For this review, take the finished solid that the model builds, in its own axes (mm). Face numbers are marked on the shaded views. A direction names the side the tool comes from. Round coordinates to 2 decimals unless told otherwise and drop trailing zeros. Write each loop counter-clockwise with the first axis right and the second up, starting at its lowest first coordinate (ties: lowest second). Pieces come first, ordered by that corner, then holes. Notation, with made-up numbers: (40, 81.25) -> (86, 81.25) arc R11 cw to (86, 97.25) -> close; hole circle Ø2 at (30, 9.5). An arc over 180 degrees is marked (long way). Answer in a Markdown table with one row per item. Add a question column.
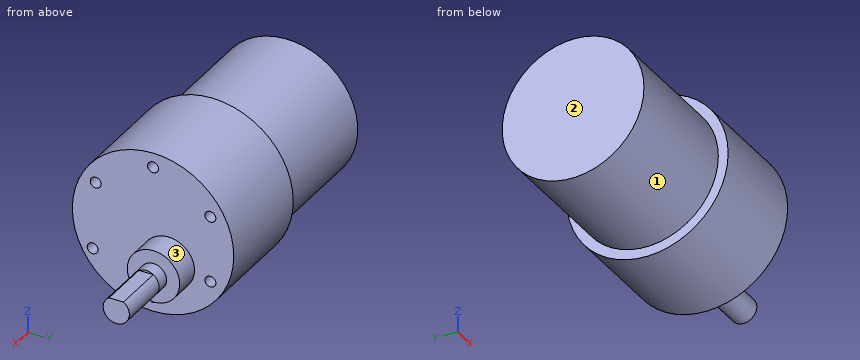
```python
from build123d import *

# Parameters (mm, degrees)
SKETCH061_R             = 16.25
PAD047_DEPTH            = 30
SKETCH062_R             = 18.5
PAD048_DEPTH            = 24
SKETCH063_R             = 1.25
POCKET012_DEPTH         = 4
SKETCH064_R             = 6
PAD049_DEPTH            = 6
SKETCH065_R             = 3
PAD050_DEPTH            = 3
PAD051_DEPTH            = 12
BODY015_ROLL_ANGLE      = -90
BODY015_PLACEMENT_ANGLE = -90


with BuildPart() as part:
    # Sketch061 → Pad047 (new body)
    with BuildSketch(Plane.XY):
        Circle(SKETCH061_R)
    extrude(amount=PAD047_DEPTH)

    # Sketch062 (on Face3 of Pad047) → Pad048 (join)
    with BuildSketch(Plane.XY.offset(30)):
        Circle(SKETCH062_R)
    extrude(amount=PAD048_DEPTH)

    # Sketch063 (on Face5 of Pad048) → Pocket012 (cut)
    with BuildSketch(Plane.XY.offset(54)):
        with Locations((-13.14747, 7.590696)):
            Circle(SKETCH063_R)
        with Locations((-13.14747, -7.590696)):
            Circle(SKETCH063_R)
        with Locations((13.14747, -7.590696)):
            Circle(SKETCH063_R)
        with Locations((0, 15.181391)):
            Circle(SKETCH063_R)
        with Locations((13.853779, 7.998483)):
            Circle(SKETCH063_R)
        with Locations((0, -15.181391)):
            Circle(SKETCH063_R)
    extrude(amount=-POCKET012_DEPTH, mode=Mode.SUBTRACT)

    # Sketch064 (on Face5 of Pocket012) → Pad049 (join)
    with BuildSketch(Plane(origin=(0, 0, 54), x_dir=(0.866025, 0.5, 0), z_dir=(0, 0, 1))):
        with Locations((0, 7)):
            Circle(SKETCH064_R)
    extrude(amount=PAD049_DEPTH)

    # Sketch065 (on Face17 of Pad049) → Pad050 (join)
    with BuildSketch(Plane.XY.offset(60)):
        with Locations((-3.5, 6.062178)):
            Circle(SKETCH065_R)
    extrude(amount=PAD050_DEPTH)

    # Sketch066 (on Face21 of Pad050) → Pad051 (join)
    with BuildSketch(Plane.XY.offset(63)):
        with BuildLine():
            Line((-5.158312, 3.562178), (-1.841688, 3.562178))
            ThreePointArc((-1.841688, 3.562178), (-3.5, 9.062178), (-5.158312, 3.562178))
        make_face()
    extrude(amount=PAD051_DEPTH)


with BuildPart() as part_1:
    # Body015 roll: moved
    add(part.part.rotate(Axis((0, 0, 0), (1, 0, 0)), BODY015_ROLL_ANGLE))


with BuildPart() as part_2:
    # Body015 placement: moved
    add(part_1.part.moved(Location((-199, 213.5, 112))).rotate(Axis((-199, 213.5, 112), (0, 0, 1)), BODY015_PLACEMENT_ANGLE))


solid = part_2.part
```
1. Clearance check with flat-ended pins moving along their axes: pin 1 Ø2 at (y, z) = (201, 119.5) entering from +X; pin 2 Ø2 at (x, z) = (-164, 100.5) entering from -Y; pin 3 Ø1 at (x, y) = (-182.5, 218.5) entering from +Z. State where each tip first meets the part, or that it passes through.
2. For L1, parallel to Z at x = -146.1, y = 213.5; L2, parallel to Z at x = -147, y = 213; L3, parallel to X at y = 201, z = 109.5, list the stretches that pass through material, from the lowest coordinate up. Write a range as [from, to].
3. We need section A-A (z = 101.5). Write out the cut boundary in (x, y).
4. We need section D-D (z = 116). Write out the cut boundary in (x, y).
5. Tool access review of the marked faces 1, 2 and 3: name each direction out of +Z, -Z, +X, -X, +Y, -Y from which nothing blocks a thin tool from reaching the whole face with its end or side.
6. We need section B-B (y = 217). Write out the cut boundary in (x, z), plus the area to 3 significant figures.
7. We need section C-C (x = -172.5). Write out the cut boundary in (y, z).
Response:
| question | item | result |
|---|---|---|
| 1 | pin 1 | x = -145 |
| 1 | pin 2 | y = 198.27 |
| 1 | pin 3 | z = 127.61 |
| 2 | L1 | [93.5, 95.57], [98.07, 125.93], [128.43, 130.5] |
| 2 | L2 | [93.51, 95.67], [97.96, 126.04], [128.33, 130.49] |
| 2 | L3 | [-199, -145] |
| 3 | outline | (-199, 201.1) -> (-169, 201.1) -> (-169, 198.27) -> (-145, 198.27) -> (-145, 212.96) -> (-139, 212.96) -> (-139, 221.04) -> (-145, 221.04) -> (-145, 228.73) -> (-169, 228.73) -> (-169, 225.9) -> (-199, 225.9) -> close |
| 4 | outline | (-199, 197.75) -> (-169, 197.75) -> (-169, 195.44) -> (-145, 195.44) -> (-145, 231.56) -> (-169, 231.56) -> (-169, 229.25) -> (-199, 229.25) -> close |
| 5 | face 1 | -X |
| 5 | face 2 | +Z, -Z, -X, +Y, -Y |
| 5 | face 3 | +X |
| 6 | outline | (-199, 96.13) -> (-169, 96.13) -> (-169, 93.83) -> (-145, 93.83) -> (-145, 99.94) -> (-139, 99.94) -> (-139, 102.94) -> (-124, 102.94) -> (-124, 108.44) -> (-136, 108.44) -> (-136, 108.94) -> (-139, 108.94) -> (-139, 111.94) -> (-145, 111.94) -> (-145, 130.17) -> (-169, 130.17) -> (-169, 127.87) -> (-199, 127.87) -> close |
| 6 | area | 1,980 mm2 |
| 7 | outline | circle Ø32.5 at (213.5, 112) |
